```python
from build123d import *

# Parameters (mm, degrees)
BOSS_EXTRUDE1_DEPTH = 2.54
SKETCH2_R           = 12.7
BOSS_EXTRUDE2_DEPTH = 5.08
SKETCH3_R           = 10.16
BOSS_EXTRUDE3_DEPTH = 2.54
SKETCH4_R           = 12.7
BOSS_EXTRUDE4_DEPTH = 2.54
SKETCH5_W           = 2.54
SKETCH5_H           = 45.72
BOSS_EXTRUDE5_DEPTH = 50.8
SKETCH6_R           = 3.81
CUT_EXTRUDE1_DEPTH  = 2.54
SKETCH6_3_R         = 3.81
CUT_EXTRUDE2_DEPTH  = 30.988
CUT_EXTRUDE3_DEPTH  = 31.988


with BuildPart() as part:
    # Sketch1 → Boss-Extrude1 (new body)
    with BuildSketch(Plane(origin=(0, 0, 0), x_dir=(1, 0, 0), z_dir=(0, 1, 0))):
        with BuildLine():
            Line((-12.954, -25.4), (12.954, -25.4))
            ThreePointArc((12.954, -25.4), (14.750051224, -24.656051224), (15.494, -22.86))
            Line((15.494, -22.86), (15.494, 22.86))
            ThreePointArc((15.494, 22.86), (14.750051224, 24.656051224), (12.954, 25.4))
            Line((12.954, 25.4), (-12.954, 25.4))
            ThreePointArc((-12.954, 25.4), (-14.750051224, 24.656051224), (-15.494, 22.86))
            Line((-15.494, 22.86), (-15.494, -22.86))
            ThreePointArc((-15.494, -22.86), (-14.750051224, -24.656051224), (-12.954, -25.4))
        make_face()
    extrude(amount=BOSS_EXTRUDE1_DEPTH)

    # Sketch2 → Boss-Extrude2 (add)
    with BuildSketch(Plane(origin=(0, 2.54, 0), x_dir=(1, 0, 0), z_dir=(0, 1, 0))):
        Circle(SKETCH2_R)
    extrude(amount=BOSS_EXTRUDE2_DEPTH)

    # Sketch3 → Boss-Extrude3 (add)
    with BuildSketch(Plane(origin=(0, 7.62, 0), x_dir=(1, 0, 0), z_dir=(0, 1, 0))):
        Circle(SKETCH3_R)
    extrude(amount=BOSS_EXTRUDE3_DEPTH)

    # Sketch4 → Boss-Extrude4 (add)
    with BuildSketch(Plane(origin=(0, 10.16, 0), x_dir=(1, 0, 0), z_dir=(0, 1, 0))):
        Circle(SKETCH4_R)
    extrude(amount=BOSS_EXTRUDE4_DEPTH)

    # Sketch5 → Boss-Extrude5 (add)
    with BuildSketch(Plane.XZ):
        with Locations((-14.224, 0)):
            Rectangle(SKETCH5_W, SKETCH5_H)
        with Locations((14.224, 0)):
            Rectangle(SKETCH5_W, SKETCH5_H)
    extrude(amount=BOSS_EXTRUDE5_DEPTH)

    # Sketch6 → Cut-Extrude1 (cut)
    with BuildSketch(Plane(origin=(15.494, 0, 0), x_dir=(0, 0, -1), z_dir=(1, 0, 0))):
        with Locations((0, -40.64)):
            Circle(SKETCH6_R)
    extrude(amount=-CUT_EXTRUDE1_DEPTH, mode=Mode.SUBTRACT)

    # Sketch6<3> → Cut-Extrude2 (cut)
    with BuildSketch(Plane(origin=(15.494, 0, 0), x_dir=(0, 0, -1), z_dir=(1, 0, 0))):
        with BuildLine():
            Line((-12.7, -40.64), (-22.86, 0))
            Line((-22.86, 0), (-22.86, -50.8))
            Line((-22.86, -50.8), (9e-09, -50.8))
            ThreePointArc((9e-09, -50.8), (-8.131967778, -47.94745973), (-12.7, -40.64))
        make_face()
        with BuildLine():
            ThreePointArc((12.7, -40.64), (8.131967785, -47.947459724), (9e-09, -50.8))
            Line((9e-09, -50.8), (22.86, -50.8))
            Line((22.86, -50.8), (22.86, 0))
            Line((22.86, 0), (12.7, -40.64))
        make_face()
        with Locations((0, -40.64)):
            Circle(SKETCH6_3_R)
    extrude(amount=-CUT_EXTRUDE2_DEPTH, mode=Mode.SUBTRACT)

    # Sketch7 → Cut-Extrude3 (cut, through all)
    with BuildSketch(Plane(origin=(15.494, 0, 0), x_dir=(0, 0, -1), z_dir=(1, 0, 0))):
        with BuildLine():
            Line((-15.682995336, -7.762642077), (-10.901798835, -26.887428081))
            ThreePointArc((-10.901798835, -26.887428081), (-10.000783897, -28.273429406), (-8.437636885, -28.811387593))
            Line((-8.437636885, -28.811387593), (8.437636885, -28.811387593))
            ThreePointArc((8.437636885, -28.811387593), (10.000783897, -28.273429406), (10.901798835, -26.887428081))
            Line((10.901798835, -26.887428081), (15.682995336, -7.762642077))
            ThreePointArc((15.682995336, -7.762642077), (15.220875198, -5.583454578), (13.218833386, -4.60660159))
            Line((13.218833386, -4.60660159), (-13.218833386, -4.60660159))
            ThreePointArc((-13.218833386, -4.60660159), (-15.220875198, -5.583454578), (-15.682995336, -7.762642077))
        make_face()
    extrude(amount=-CUT_EXTRUDE3_DEPTH, mode=Mode.SUBTRACT)


solid = part.part
```
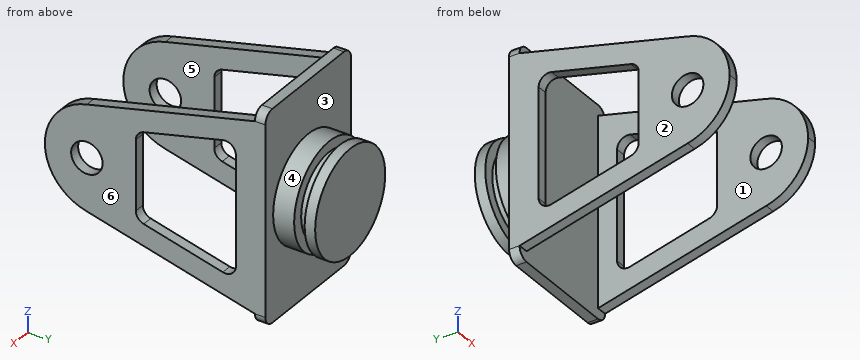
Source: CAD feature listing. Evaluate the final solid. Frame: model axes, mm. Face numbers are marked on the shaded views. A direction names the side the tool comes from. Coordinates: 2 decimals unless noted, no trailing zeros. Loops run counter-clockwise (first coordinate to the right, second up) from the corner with the lowest first, then second, coordinate; pieces in that order, holes last. Notation, with made-up numbers: (49, -25) - (78, -25) arc R27 ccw to (78, 13) - close; hole circle Ø5 at (6.5, 60). An arc over 180 degrees is marked (long way). Answer as CSV lines item,"result".
1. Reachability of the marked faces 1, 2 and 3 from +Z, -Z, +X, -X, +Y, -Y: full face, straight path, thin tool, end or side. Return the list, or none.
Established:
face 1,"+Z, -Z, -Y"
face 2,"+Z, -Z, -X, +Y, -Y"
face 3,"+Y"
2. Section D-D (x = -11.5). Return loops of the section in (y, z).
Established:
outline,"(0, -25.4) - (2.54, -25.4) - (2.54, -5.39) - (7.62, -5.39) - (7.62, 5.39) - (2.54, 5.39) - (2.54, 25.4) - (0, 25.4) - close; (10.16, -5.39) - (12.7, -5.39) - (12.7, 5.39) - (10.16, 5.39) - close"
3. Mould query, pull axis X, two halves, no side actions, for the marked faces 4, 5 and 6. Classes: released by +X, released by -X, zero draft, split by the parting line, or undercut.
Established:
face 4,"split by the parting line"
face 5,"undercut"
face 6,"released by +X"
4. Contact query for flat-ended pins moving along their axis: pin 1 (0.8 mm diameter, centred on x = 14.5, z = -5.5, fed in from -Y); pin 2 (7.5 mm diameter, centred on x = -5.5, z = 3.5, fed in from -Y); pin 3 (3 mm diameter, centred on x = -7.5, z = -13.5, fed in from +Y). Output: stop coordinate, or through.
Established:
pin 1,"stops at y = -49.76"
pin 2,"stops at y = 0"
pin 3,"stops at y = 2.54"
5. Section A-A (z = 18.5). Return loops of the section in (x, y), then the cut area to 3 significant figures.
Established:
outline,"(-15.49, -17.44) - (-12.95, -17.44) - (-12.95, 0) - (12.95, 0) - (12.95, -17.44) - (15.49, -17.44) - (15.49, 2.54) - (-15.49, 2.54) - close"
area,"167 mm2"
6. Section C-C (z = 12). Return loops of the section in (x, y).
Established:
outline,"(-15.49, -42.83) - (-12.95, -42.83) - (-12.95, -22.49) - (-15.49, -22.49) - close; (-15.49, -4.61) - (-12.95, -4.61) - (-12.95, 0) - (12.95, 0) - (12.95, -4.61) - (15.49, -4.61) - (15.49, 2.54) - (4.16, 2.54) - (4.16, 7.62) - (-4.16, 7.62) - (-4.16, 2.54) - (-15.49, 2.54) - close; (-4.16, 10.16) - (4.16, 10.16) - (4.16, 12.7) - (-4.16, 12.7) - close; (12.95, -42.83) - (15.49, -42.83) - (15.49, -22.49) - (12.95, -22.49) - close"
7. Section B-B (y = -35.5). Return loops of the section in (x, z) (3 decimals), then the cut area to 3 significant figures.
Established:
outline,"(-15.494, -13.985) - (-12.954, -13.985) - (-12.954, 13.985) - (-15.494, 13.985) - close; (12.954, -13.985) - (15.494, -13.985) - (15.494, 13.985) - (12.954, 13.985) - close"
area,"142 mm2"
8. Ray query, line 1 (Y direction, x = -13.45, z = 0); line 2 (X direction, y = -37.5, z = 10); line 3 (Y direction, x = 2.5, z = 12). Return the intervals inside material, ascending.
Established:
line 1,"y = -50.8 to -44.45, -36.83 to -28.81, -4.61 to 2.54"
line 2,"x = -15.49 to -12.95, 12.95 to 15.49"
line 3,"y = 0 to 7.62, 10.16 to 12.7"
